Design review of the part shown in the three views and the two pictorial views. Dimensions are in mm from the part's minimum x, y and z. A direction names the side the tool comes from. Give positions to 0.01 mm unless a question says otherwise; leave off trailing zeros. Order: outer loops, then holes, each group sorted by start corner. A loop starts at its lowest first (then second) coordinate and runs counter-clockwise, first axis right, second up. Notation, with made-up numbers: (17.5, -17.5) -> (31.5, -17.5) arc R18 cw to (31.5, 11.5) -> close; hole circle Ø4 at (11.25, -32). An arc over 180 degrees is marked (long way). Use one line per item in the form item = value.
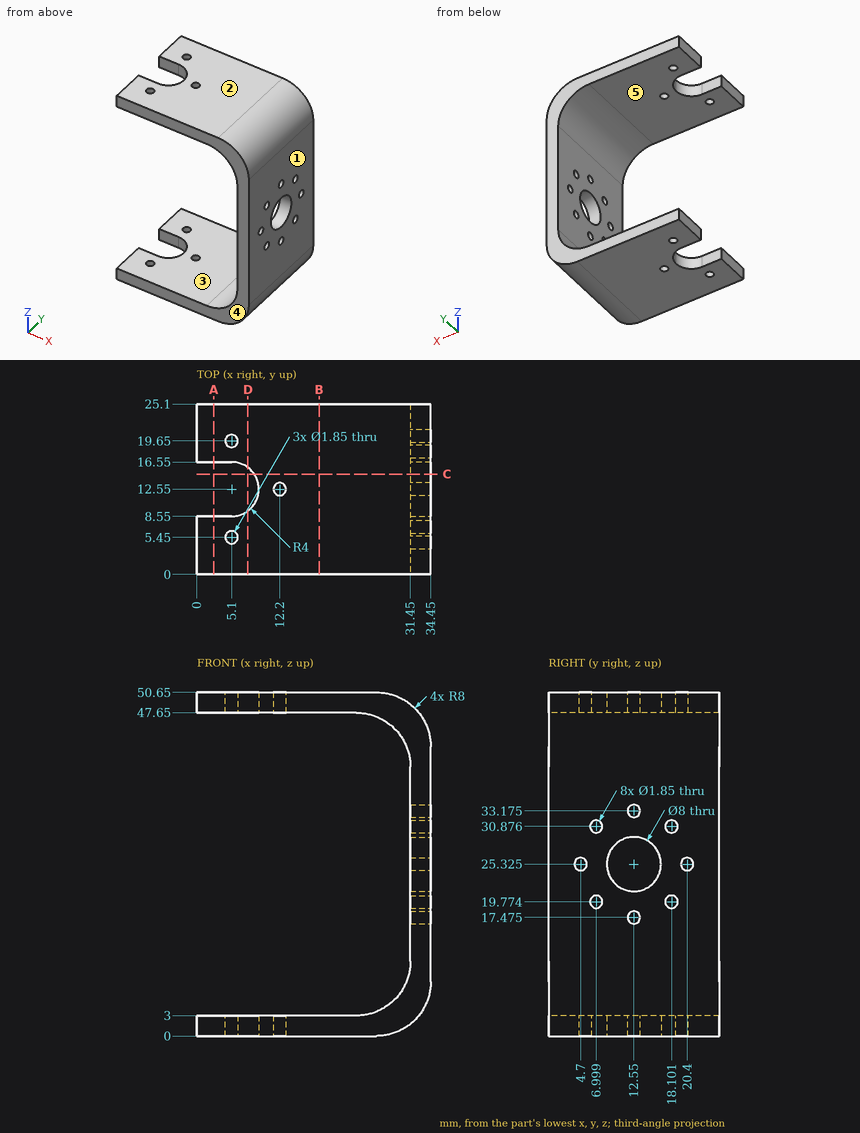
1. Add section A-A on x = 2.5. Give the boundary of the cut face in (y, z), then the cut area to 3 significant figures.
Values:
outline = (0, 0) -> (8.55, 0) -> (8.55, 3) -> (0, 3) -> close; (0, 47.65) -> (8.55, 47.65) -> (8.55, 50.65) -> (0, 50.65) -> close; (16.55, 0) -> (25.1, 0) -> (25.1, 3) -> (16.55, 3) -> close; (16.55, 47.65) -> (25.1, 47.65) -> (25.1, 50.65) -> (16.55, 50.65) -> close
area = 103 mm^2
2. Tool access review of the marked faces 4 and 5: name each direction out of +Z, -Z, +X, -X, +Y, -Y from which nothing blocks a thin tool from reaching the whole face with its end or side.
Values:
face_4 = +Z, -Z, +X, -X, -Y
face_5 = -X, +Y, -Y
3. For L1, parallel to Z at x = 19, y = 5.5; L2, parallel to Y at x = 12.2, z = 1.8 (3 decimals); L3, parallel to X at y = 6.75, z = 13.5, list the stretches that pass through material, from the lowest coordinate up.
Values:
L1 = 0 to 3, 47.65 to 50.65
L2 = 0 to 11.625, 13.475 to 25.1
L3 = 31.45 to 34.45
4. Add section D-D on x = 7.5. Give the boundary of the cut face in (y, z), then the cut area to 3 significant figures.
Values:
outline = (0, 0) -> (9.35, 0) -> (9.35, 3) -> (0, 3) -> close; (0, 47.65) -> (9.35, 47.65) -> (9.35, 50.65) -> (0, 50.65) -> close; (15.75, 0) -> (25.1, 0) -> (25.1, 3) -> (15.75, 3) -> close; (15.75, 47.65) -> (25.1, 47.65) -> (25.1, 50.65) -> (15.75, 50.65) -> close
area = 112 mm^2
5. The part is to be moulded in two halves that separate along Z. For the marked faces 1, 2 and 3, say which applies: +Z half, -Z half, draft (parallel to the pull), parting line (faces both ways), or undercut.
Values:
face_1 = draft
face_2 = +Z half
face_3 = undercut
6. For pin 1 Ø1.1 at (y, z) = (20.4, 25.325) entering from -X; pin 2 Ø2.5 at (y, z) = (7, 30.88) entering from -X, all flat-tipped, find the tip position at first contact; note any pin that passes through.
Values:
pin_1 = through
pin_2 = 31.45
7. Add section C-C on y = 14.75. Give the boundary of the cut face in (x, z), then the cut area to 3 significant figures.
Values:
outline = (8.44, 0) -> (26.45, 0) arc R8 ccw to (34.45, 8) -> (34.45, 21.98) -> (31.45, 21.98) -> (31.45, 11) arc R8 cw to (23.45, 3) -> (8.44, 3) -> close; (8.44, 47.65) -> (23.45, 47.65) arc R8 cw to (31.45, 39.65) -> (31.45, 28.67) -> (34.45, 28.67) -> (34.45, 42.65) arc R8 ccw to (26.45, 50.65) -> (8.44, 50.65) -> close
area = 270 mm^2
8. Add section B-B on x = 18. Give the boundary of the cut face in (y, z), then the cut area to 3 significant figures.
Values:
outline = (0, 0) -> (25.1, 0) -> (25.1, 3) -> (0, 3) -> close; (0, 47.65) -> (25.1, 47.65) -> (25.1, 50.65) -> (0, 50.65) -> close
area = 151 mm^2
